Geometry: see drawing. Coordinates: mm, zero at the bounding-box minimum. Coordinates: 2 decimals unless noted, no trailing zeros. Loops run counter-clockwise (first coordinate to the right, second up) from the corner with the lowest first, then second, coordinate; pieces in that order, holes last. Notation, with made-up numbers: (19.25, -7.5) -> (66.25, -7.5) arc R10 cw to (66.25, 1.5) -> close; hole circle Ø3 at (-2, -18.75). An arc over 180 degrees is marked (long way). One line per item, written item: value. Start each with the question number.
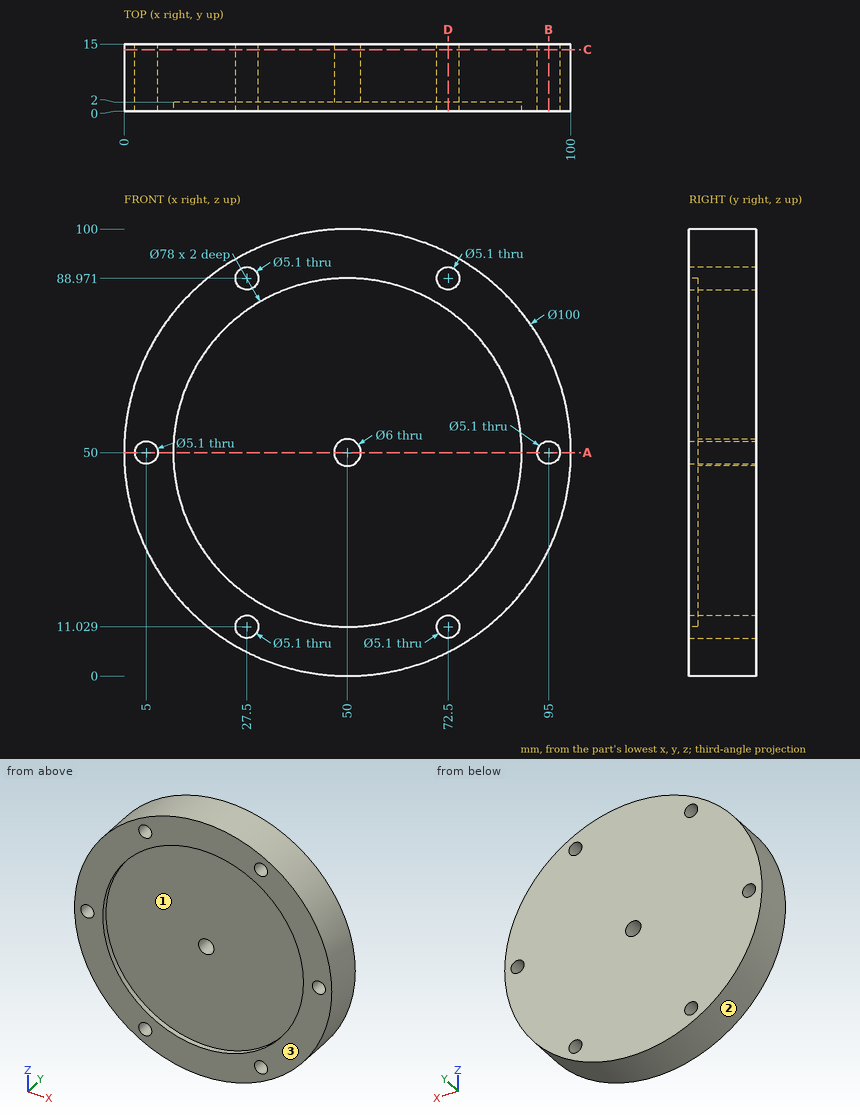
1. Section B-B on x = 95. Return the cut outline in (y, z).
2. Pin query (flat end, axial travel): pin 1 Ø5 at (x, y) = (51.5, 2) entering from +Z; pin 2 Ø8 at (y, z) = (11.5, 68) entering from -X; pin 3 Ø1 at (x, z) = (66, 21) entering from -Y. Return the tip coordinate at first contact, or that it passes through.
3. Section D-D on x = 72.5. Return the cut outline in (y, z) (1 decimal), plus the area to 3 significant figures.
4. Section C-C on y = 13.75. Return the cut outline in (x, z).
5. Line query: L1, parallel to X at y = 13, z = 11; L2, parallel to Z at x = 74.5, y = 3; L3, parallel to Z at x = 72.5, y = 11. Output: solid intervals per line, ascending. Write a range as [from, to].
6. Draft query along Z for the marked faces 1, 2 and 3. Return one class per face: released by +Z, released by -Z, zero draft, split by the parting line, or undercut.
7. Section A-A on z = 50. Return the cut outline in (x, y).
Checks:
1. outline: (0, 28.21) -> (15, 28.21) -> (15, 47.45) -> (0, 47.45) -> close; (0, 52.55) -> (15, 52.55) -> (15, 71.79) -> (0, 71.79) -> close
2. pin 1: z = 100
2. pin 2: x = 2
2. pin 3: y = 2
3. outline: (0, 5.3) -> (15, 5.3) -> (15, 8.5) -> (0, 8.5) -> close; (0, 13.6) -> (15, 13.6) -> (15, 86.4) -> (0, 86.4) -> (0, 81.9) -> (2, 81.9) -> (2, 18.1) -> (0, 18.1) -> close; (0, 91.5) -> (15, 91.5) -> (15, 94.7) -> (0, 94.7) -> close
3. area: 1,060 mm²
4. outline: circle Ø100 at (50, 50); hole circle Ø5.1 at (5, 50); hole circle Ø5.1 at (27.5, 11.03); hole circle Ø5.1 at (27.5, 88.97); hole circle Ø6 at (50, 50); hole circle Ø5.1 at (72.5, 11.03); hole circle Ø5.1 at (72.5, 88.97); hole circle Ø5.1 at (95, 50)
5. L1: [18.71, 24.95], [30.05, 69.95], [75.05, 81.29]
5. L2: [6.41, 9.45], [12.61, 87.39], [90.55, 93.59]
5. L3: [5.35, 8.48], [13.58, 86.42], [91.52, 94.65]
6. face 1: undercut
6. face 2: split by the parting line
6. face 3: zero draft
7. outline: (0, 0) -> (2.45, 0) -> (2.45, 15) -> (0, 15) -> close; (7.55, 0) -> (11, 0) -> (11, 2) -> (47, 2) -> (47, 15) -> (7.55, 15) -> close; (53, 2) -> (89, 2) -> (89, 0) -> (92.45, 0) -> (92.45, 15) -> (53, 15) -> close; (97.55, 0) -> (100, 0) -> (100, 15) -> (97.55, 15) -> close
